Input: part model. Units: mm. Frame: model coordinates. A direction names the side the tool comes from. Round coordinates to 2 decimals unless told otherwise and drop trailing zeros. Loops run counter-clockwise (first coordinate to the right, second up) from the corner with the lowest first, then second, coordinate; pieces in that order, holes last.
1) Ray query, line 1 along X through (y, z) = (38, 39); line 2 along Y through (x, z) = (67, 2); line 3 along Y through (x, z) = (25.4, 34.75). Return the intervals inside material, ascending.
2) Section D-D, the plane z = 41.5. Return loops of the section in (x, y), and give its area (3 significant figures).
3) Draft query along Y for faces 1 (the face through (76, 70, 0)), 2 (the face through (61, 76.2, 31)), 3 (the face through (76, 63.5, 6)). Return one class per face: pulls with the +Y half, pulls with the -Y half, needs draft (parallel to the pull), parting line crosses it, or undercut.
4) Access query for faces 4 (the face through (36, 47, 25.4)), 5 (the face through (0, 38, 38)), 6 (the face through (76, 38, 12.7)). Directions: +Z, -Z, +X, -X, +Y, -Y. A direction counts if a zero-diameter tool reaches every point of the face in a straight line with its end or side. Return the directions, or none.
5) First-contact query: pin 1 (23 mm diameter, centred on x = 25.4, y = 38.1, fed in from +Z); pin 2 (12.5 mm diameter, centred on y = 30, z = 17, fed in from -X). Flat tips, straight axial feed; report the tip coordinate or a pass-through.
6) Section A-A, the plane z = 4.5. Return loops of the section in (x, y).
7) Section B-B, the plane x = 25.4. Return loops of the section in (y, z), and give its area (3 significant figures).
8) Section C-C, the plane y = 38.1. Return loops of the section in (x, z), and give its area (3 significant figures).
from build123d import *

# Parameters (mm, degrees)
F5_W      = 101.6
F5_H      = 76.2
F6_DEPTH  = 50.8
F7_W      = 50.8
F7_H      = 76.2
F8_DEPTH  = 25.4
F9_R      = 12.7
F10_DEPTH = 76.2
F12_DEPTH = 12.7


with BuildPart() as f6:
    # F5 (on Top) → F6 (new body)
    with BuildSketch(Plane.XY):
        with Locations((50.8, 38.1)):
            Rectangle(F5_W, F5_H)
    extrude(amount=F6_DEPTH)

    # F7 (on Top) → F8 (cut)
    with BuildSketch(Plane.XY):
        with Locations((25.4, 38.1)):
            Rectangle(F7_W, F7_H)
    extrude(amount=F8_DEPTH, mode=Mode.SUBTRACT)

    # F9 (on Top) → F10 (cut)
    with BuildSketch(Plane.XY):
        with Locations((25.4, 38.1)):
            Circle(F9_R)
    extrude(amount=F10_DEPTH, mode=Mode.SUBTRACT)

    # F11 (on face) → F12 (cut)
    with BuildSketch(Plane(origin=(0, 0, 0), x_dir=(1, 0, 0), z_dir=(0, 0, -1))):
        Polygon((101.6, -12.7), (83.254352, -12.7), (50.8, -12.7), (50.8, -63.5), (101.6, -63.5), align=None)
    extrude(amount=-F12_DEPTH, mode=Mode.SUBTRACT)


solid = f6.part
Final values:
1. line 1: x = 0 to 12.7, 38.1 to 101.6
1. line 2: y = 0 to 12.7, 63.5 to 76.2
1. line 3: y = 0 to 25.4, 50.8 to 76.2
2. outline: (0, 0) - (101.6, 0) - (101.6, 76.2) - (0, 76.2) - close; hole circle Ø25.4 at (25.4, 38.1)
2. area: 7,240 mm2
3. face 1: needs draft
3. face 2: pulls with the +Y half
3. face 3: undercut
4. face 4: -Z, -X, +Y, -Y
4. face 5: +Z, -Z, -X, +Y, -Y
4. face 6: -Z, +X, -X
5. pin 1: passes through
5. pin 2: stops at x = 50.8
6. outline: (50.8, 0) - (101.6, 0) - (101.6, 12.7) - (50.8, 12.7) - close; (50.8, 63.5) - (101.6, 63.5) - (101.6, 76.2) - (50.8, 76.2) - close
7. outline: (0, 25.4) - (25.4, 25.4) - (25.4, 50.8) - (0, 50.8) - close; (50.8, 25.4) - (76.2, 25.4) - (76.2, 50.8) - (50.8, 50.8) - close
7. area: 1,290 mm2
8. outline: (0, 25.4) - (12.7, 25.4) - (12.7, 50.8) - (0, 50.8) - close; (38.1, 25.4) - (50.8, 25.4) - (50.8, 12.7) - (101.6, 12.7) - (101.6, 50.8) - (38.1, 50.8) - close
8. area: 2,580 mm2
